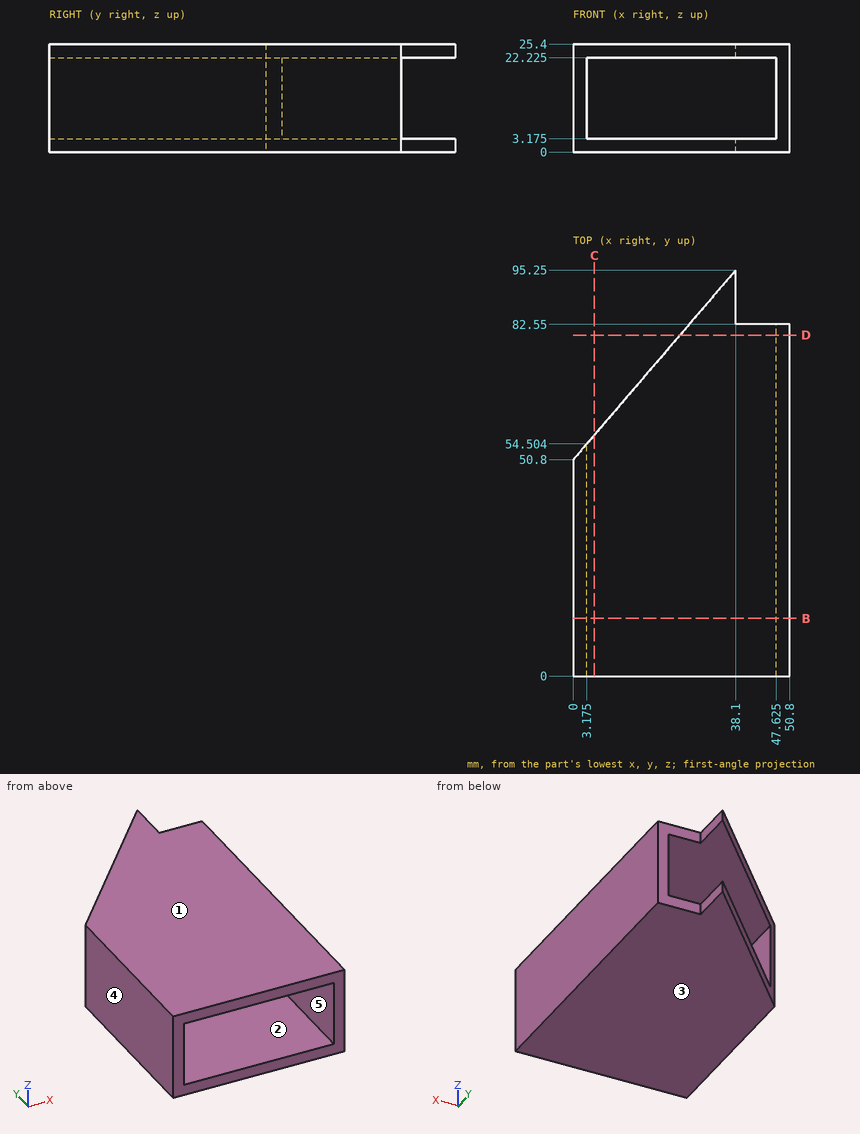
Print and shaded views of the part. All mm, measured from the part's lowest x, y and z. A direction names the side the tool comes from. Coordinates: 2 decimals unless noted, no trailing zeros. Order: outer loops, then holes, each group sorted by start corner. A loop starts at its lowest first (then second) coordinate and runs counter-clockwise, first axis right, second up. Notation, with made-up numbers: (-26.5, 31) - (-5.5, 31) arc R9 ccw to (-5.5, 44) - close; hole circle Ø11 at (82, -19). An arc over 180 degrees is marked (long way). Return JSON: item names as keys, results as strings. Group by question number.
Item 1: Pin check, flat tips, straight feed: pin 1 (1.6 mm diameter, centred on y = 92, z = 2, fed in from +X); pin 2 (13.5 mm diameter, centred on x = 26, y = 46, fed in from -Z); pin 3 (10 mm diameter, centred on x = 26.5, z = 9.5, fed in from +Y); pin 4 (14 mm diameter, centred on x = 41.5, z = 13.5, fed in from +Y). Stop position of each tip, or through.
Item 2: Cut at D-D (y = 80). List the corners of the cut face in (x, z) (1 decimal), plus the area to 3 significant figures.
Item 3: Cut at B-B (y = 13.5). List the corners of the cut face in (x, z) (3 decimals).
Item 4: Pull direction X, two halves, no side cores. Call the marked faces 3, 4 and 5: pulls with the +X half, pulls with the -X half, needs draft (parallel to the pull), parting line crosses it, or undercut.
Item 5: Which spindle directions (+Z, -Z, +X, -X, +Y, -Y) get a long thin tool onto all of the face, cutting with end or side? Do the marked faces 1 and 2. Say none if no direction does.
Item 6: Drill centre lines: probe 1 along X at (y, z) = (42, 17.25) (3 decimals); probe 2 along Z at (x, y) = (31, 46.5) (3 decimals); probe 3 along X at (y, z) = (57.5, 10) (3 decimals). Where is each one in solid material? Low to high. Write a range as from..to.
Item 7: Cut at C-C (x = 5). List the corners of the cut face in (y, z) (1 decimal), plus the area to 3 significant figures.
Check values:
{
 "1": {"pin 1": "stops at x = 38.1", "pin 2": "stops at z = 0", "pin 3": "passes through", "pin 4": "stops at y = 82.55"},
 "2": {"outline": "(25, 0) - (50.8, 0) - (50.8, 25.4) - (25, 25.4) - (25, 22.2) - (47.6, 22.2) - (47.6, 3.2) - (25, 3.2) - close", "area": "224 mm2"},
 "3": {"outline": "(0, 0) - (50.8, 0) - (50.8, 25.4) - (0, 25.4) - close; hole (3.175, 3.175) - (47.625, 3.175) - (47.625, 22.225) - (3.175, 22.225) - close"},
 "4": {"face 3": "needs draft", "face 4": "pulls with the -X half", "face 5": "undercut"},
 "5": {"face 1": "+Z, +X, -X, +Y, -Y", "face 2": "+Y, -Y"},
 "6": {"probe 1": "x = 0..3.175, 47.625..50.8", "probe 2": "z = 0..3.175, 22.225..25.4", "probe 3": "x = 47.625..50.8"},
 "7": {"outline": "(0, 0) - (56.6, 0) - (56.6, 3.2) - (0, 3.2) - close; (0, 22.2) - (56.6, 22.2) - (56.6, 25.4) - (0, 25.4) - close", "area": "360 mm2"}
}
